Work out the finished part from the listing and answer in its coordinate system (mm). A direction names the side the tool comes from. Coordinates: 2 decimals unless noted, no trailing zeros. Loops run counter-clockwise (first coordinate to the right, second up) from the corner with the lowest first, then second, coordinate; pieces in that order, holes last. Notation, with made-up numbers: (-10.75, -35.75) -> (9.25, -35.75) arc R16 ccw to (9.25, -10.75) -> close; hole circle Ø2 at (30, 43.25). An arc over 180 degrees is marked (long way). Answer as CSV lines item,"result".
```python
from build123d import *

# Parameters (mm, degrees)
BOSS_EXTRUDE1_DEPTH = 2
BOSS_EXTRUDE2_DEPTH = 1.5
SKETCH4_W           = 1.550075991
SKETCH4_H           = 4.899134607
BOSS_EXTRUDE3_DEPTH = 1
CHAMFER1_SIZE       = 0.2
CUT_EXTRUDE1_START  = -2
SKETCH5_W           = 3.300200616
SKETCH5_H           = 1
SKETCH5_W_2         = 3.300200617
CUT_EXTRUDE1_DEPTH  = 2
SKETCH6_W           = 2
SKETCH6_H           = 6.999134607
BOSS_EXTRUDE4_DEPTH = 2


with BuildPart() as part:
    # Sketch2 → Boss-Extrude1 (new body)
    with BuildSketch(Plane.XY):
        Polygon((285.431409328, 90.45473243), (277.431409328, 90.45473243), (277.431409328, 89.55473243), (274.231409328, 89.55473243), (274.231409328, 84.955597823), (273.006316619, 84.955597823), (273.006316619, 87.985794184), (266.055906266, 87.985794184), (266.055906266, 84.955597823), (264.955830275, 84.955597823), (264.955830275, 91.95473243), (297.906988381, 91.95473243), (297.906988381, 84.955597823), (296.80691239, 84.955597823), (296.80691239, 87.985794184), (289.856502038, 87.985794184), (289.856502038, 84.955597823), (288.631409328, 84.955597823), (288.631409328, 89.55473243), (285.431409328, 89.55473243), align=None)
    extrude(amount=-BOSS_EXTRUDE1_DEPTH)

    # Sketch3 → Boss-Extrude2 (add)
    with BuildSketch(Plane.XY):
        Polygon((274.231409328, 89.45473243), (264.955830275, 89.45473243), (264.955830275, 84.955597823), (266.055906266, 84.955597823), (266.055906266, 87.985794184), (273.006316619, 87.985794184), (273.006316619, 84.955597823), (274.231409328, 84.955597823), align=None)
        Polygon((297.906988381, 89.45473243), (288.631409328, 89.45473243), (288.631409328, 84.955597823), (289.856502038, 84.955597823), (289.856502038, 87.985794184), (296.80691239, 87.985794184), (296.80691239, 84.955597823), (297.906988381, 84.955597823), align=None)
    extrude(amount=BOSS_EXTRUDE2_DEPTH)

    # Sketch4 → Boss-Extrude3 (add)
    with BuildSketch(Plane.XY.offset(1.5)):
        with Locations((265.280868271, 87.405165127)):
            Rectangle(SKETCH4_W, SKETCH4_H)
        with Locations((297.581950386, 87.405165127)):
            Rectangle(SKETCH4_W, SKETCH4_H)
    extrude(amount=BOSS_EXTRUDE3_DEPTH)

    # Chamfer1
    chamfer1_edges = [part.edges().sort_by_distance(p)[0] for p in [
        (264.505830275, 87.405165127, 1.5),
        (265.280868271, 89.85473243, 1.5),
        (298.356988381, 87.405165127, 1.5),
        (297.581950386, 89.85473243, 1.5),
    ]]
    chamfer(chamfer1_edges, length=CHAMFER1_SIZE)

    # Sketch5 → Cut-Extrude1 (cut)
    with BuildSketch(Plane(origin=(0, 0, -2), x_dir=(-1, 0, 0), z_dir=(0, 0, -1)).offset(CUT_EXTRUDE1_START)):
        with Locations((-269.530111382, 88.485794184)):
            Rectangle(SKETCH5_W, SKETCH5_H)
        with Locations((-293.332707275, 88.485794184)):
            Rectangle(SKETCH5_W_2, SKETCH5_H)
    extrude(amount=CUT_EXTRUDE1_DEPTH, mode=Mode.SUBTRACT)

    # Sketch6 → Boss-Extrude4 (add)
    with BuildSketch(Plane(origin=(0, 0, -2), x_dir=(-1, 0, 0), z_dir=(0, 0, -1))):
        with Locations((-298.906988381, 88.455165127)):
            Rectangle(SKETCH6_W, SKETCH6_H)
        with Locations((-263.955830275, 88.455165127)):
            Rectangle(SKETCH6_W, SKETCH6_H)
    extrude(amount=-BOSS_EXTRUDE4_DEPTH)


solid = part.part
```
(1) Flat-ended cylindrical pins translate along their axes: pin 1 Ø2 at (x, z) = (293, -0.5) entering from -Y; pin 2 Ø0.9 at (x, z) = (265.5, 2) entering from +Y; pin 3 Ø1.2 at (x, z) = (292.5, 1) entering from +Y. Find the tip coordinate at first contact, or state that the pin passes through.
Computed values:
pin 1,"y = 87.99"
pin 2,"y = 89.85"
pin 3,"y = 89.45"
(2) A cutting plane is placed at C-C, the plane y = 86. Write down the section's boundary in (x, z).
Computed values:
outline,"(262.96, -2) -> (266.06, -2) -> (266.06, 2.5) -> (264.51, 2.5) -> (264.51, 1.7) -> (264.71, 1.5) -> (264.96, 1.5) -> (264.96, 0) -> (262.96, 0) -> close; (273.01, -2) -> (274.23, -2) -> (274.23, 1.5) -> (273.01, 1.5) -> close; (288.63, -2) -> (289.86, -2) -> (289.86, 1.5) -> (288.63, 1.5) -> close; (296.81, -2) -> (299.91, -2) -> (299.91, 0) -> (297.91, 0) -> (297.91, 1.5) -> (298.16, 1.5) -> (298.36, 1.7) -> (298.36, 2.5) -> (296.81, 2.5) -> close"
(3) Which of the six approach directions +Z, -Z, +X, -X, +Y, -Y give full straight-line access (tool end or side, diameter ignored) to faces 3 (the face through (298, 84.956, -0.3)), 4 (the face through (281, 90.455, -1)), 5 (the face through (291.683, 88.5, -1)), 6 (the face through (298, 89.855, 2)), 7 (the face through (291.8, 88.2, 1.5))?
Computed values:
face 3,"+Z, -Z, +X, -X, -Y"
face 4,"+Z, -Z, -Y"
face 5,"-Z, -Y"
face 6,"+Z, +X, -X, +Y"
face 7,"+Z, +Y, -Y"
(4) Consider line 1 along X through (y, z) = (88.25, -1.4); line 2 along X through (y, z) = (85.5, 1.2); line 3 along X through (y, z) = (88.25, 0.05). Determine where each line is inside the solid, lowest interval first.
Computed values:
line 1,"262.96 to 267.88, 271.18 to 274.23, 288.63 to 291.68, 294.98 to 299.91"
line 2,"264.96 to 266.06, 273.01 to 274.23, 288.63 to 289.86, 296.81 to 297.91"
line 3,"264.96 to 274.23, 288.63 to 297.91"
(5) A cutting plane is placed at B-B, the plane z = 0.8. Write down the section's boundary in (x, y).
Computed values:
outline,"(264.96, 84.96) -> (266.06, 84.96) -> (266.06, 87.99) -> (273.01, 87.99) -> (273.01, 84.96) -> (274.23, 84.96) -> (274.23, 89.45) -> (264.96, 89.45) -> close; (288.63, 84.96) -> (289.86, 84.96) -> (289.86, 87.99) -> (296.81, 87.99) -> (296.81, 84.96) -> (297.91, 84.96) -> (297.91, 89.45) -> (288.63, 89.45) -> close"
(6) A cutting plane is placed at D-D, the plane x = 294. Write down the section's boundary in (y, z).
Computed values:
outline,"(87.99, 0) -> (88.99, 0) -> (88.99, -2) -> (91.95, -2) -> (91.95, 0) -> (89.45, 0) -> (89.45, 1.5) -> (87.99, 1.5) -> close"
(7) For a pull along X with two mould halves and no side action, classify faces 1 (the face through (294.983, 88.5, -1)), 2 (the face through (298, 87, 2.5)) as pulls with the +X half, pulls with the -X half, needs draft (parallel to the pull), parting line crosses it, or undercut.
Computed values:
face 1,"undercut"
face 2,"needs draft"
